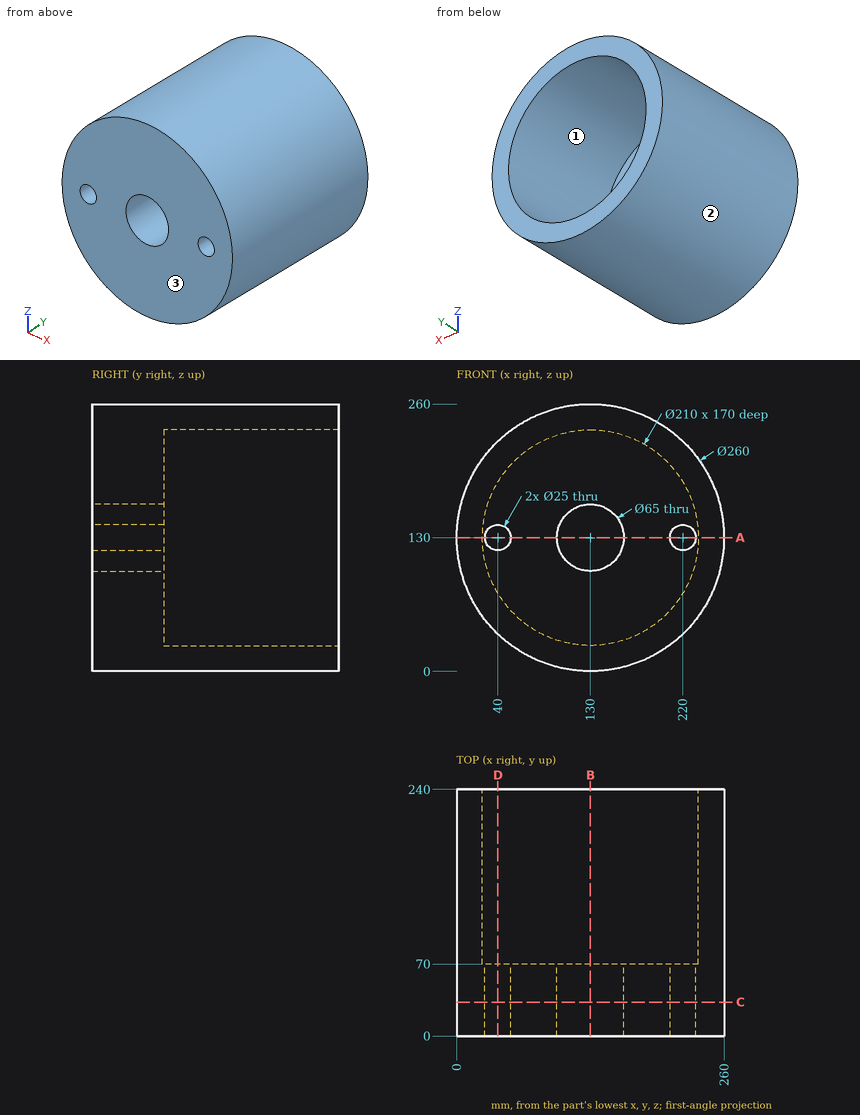
Source: three-view drawing plus pictorial views. Frame: mm from the lowest corner of the part. Give positions to 0.01 mm unless a question says otherwise; leave off trailing zeros. Order: outer loops, then holes, each group sorted by start corner. A loop starts at its lowest first (then second) coordinate and runs counter-clockwise, first axis right, second up. Notation, with made-up numbers: M -24,74 L 25,74 A19 ccw 25,102 Z; hole C 82,20 d4. An arc over 180 degrees is marked long. Return JSON: item names as keys, results as strings.
1) Line query: L1, parallel to X at y = 17, z = 130; L2, parallel to Y at x = 99, z = 215.5; L3, parallel to Z at x = 170, y = 230.5. Output: solid intervals per line, ascending. Write a range as [from, to].
Taken from the geometry:
{"L1": "x = [0, 27.5], [52.5, 97.5], [162.5, 207.5], [232.5, 260]", "L2": "y = [0, 70]", "L3": "z = [6.31, 32.92], [227.08, 253.69]"}
2) Section query B-B on x = 130. Output: boundary loops of the cut face in (y, z), and give its area (4 significant figures).
Taken from the geometry:
{"outline": "M 0,0 L 240,0 L 240,25 L 70,25 L 70,97.5 L 0,97.5 Z; M 0,162.5 L 70,162.5 L 70,235 L 240,235 L 240,260 L 0,260 Z", "area": "22,150 mm2"}
3) Contact query for flat-ended pins moving along their axis: pin 1 (1 mm diameter, centred on x = 229.5, y = 32.5, fed in from -Z); pin 2 (10 mm diameter, centred on y = 160.5, z = 74.5, fed in from +X); pin 3 (6 mm diameter, centred on x = 67.5, y = 52, fed in from +Z). Output: stop coordinate, or through.
Taken from the geometry:
{"pin 1": "stops at z = 45.74", "pin 2": "stops at x = 249.79", "pin 3": "stops at z = 245.58"}
4) Section query D-D on x = 40. Output: boundary loops of the cut face in (y, z).
Taken from the geometry:
{"outline": "M 0,36.19 L 240,36.19 L 240,75.92 L 70,75.92 L 70,117.5 L 0,117.5 Z; M 0,142.5 L 70,142.5 L 70,184.08 L 240,184.08 L 240,223.81 L 0,223.81 Z"}
5) Mould query, pull axis X, two halves, no side actions, for the marked faces 1, 2 and 3. Classes: released by +X, released by -X, zero draft, split by the parting line, or undercut.
Taken from the geometry:
{"face 1": "undercut", "face 2": "split by the parting line", "face 3": "zero draft"}
6) Section query A-A on z = 130. Output: boundary loops of the cut face in (x, y), and give its area (4 significant figures).
Taken from the geometry:
{"outline": "M 0,0 L 27.5,0 L 27.5,70 L 25,70 L 25,240 L 0,240 Z; M 52.5,0 L 97.5,0 L 97.5,70 L 52.5,70 Z; M 162.5,0 L 207.5,0 L 207.5,70 L 162.5,70 Z; M 232.5,0 L 260,0 L 260,240 L 235,240 L 235,70 L 232.5,70 Z", "area": "18,650 mm2"}
7) Section query C-C on y = 33. Output: boundary loops of the cut face in (x, z).
Taken from the geometry:
{"outline": "C 130,130 d260; hole C 40,130 d25; hole C 130,130 d65; hole C 220,130 d25"}
